```python
from build123d import *

# Parameters (mm, degrees)
F0_W     = 24
F0_H     = 24
F1_DEPTH = 120
F2_R     = 8.3
F3_DEPTH = 250
F4_W     = 28.767977
F4_H     = 14
F4_W_2   = 2.367542
F4_W_3   = 2.400435
F4_W_4   = 24
F5_DEPTH = 250


with BuildPart() as f1:
    # F0 (on Front) → F1 (new body)
    with BuildSketch(Plane.XZ):
        with Locations((-6.988064, 12)):
            Rectangle(F0_W, F0_H)
    extrude(amount=F1_DEPTH)

    # F2 (on face) → F3 (cut)
    with BuildSketch(Plane.XZ.offset(120)):
        with Locations((-6.988064, 0)):
            Circle(F2_R)
    extrude(amount=-F3_DEPTH, mode=Mode.SUBTRACT)

    # F4 (on face) → F5 (cut)
    with BuildSketch(Plane.XZ.offset(120)):
        with Locations((-7.004511, 17)):
            Rectangle(F4_W, F4_H)
        with Locations((6.195707, 17)):
            Rectangle(F4_W_2, F4_H)
        with Locations((-20.188281, 17)):
            Rectangle(F4_W_3, F4_H)
        with Locations((-6.988064, 17)):
            Rectangle(F4_W_4, F4_H)
    extrude(amount=-F5_DEPTH, mode=Mode.SUBTRACT)


solid = f1.part
```
Part model, mm, in its own coordinate system. Round coordinates to 2 decimals unless told otherwise and drop trailing zeros. Loops run counter-clockwise (first coordinate to the right, second up) from the corner with the lowest first, then second, coordinate; pieces in that order, holes last.
Item 1: Cut at B-B, the plane y = -52. Give the cut face in (x, z).
Item 2: Drill centre lines: line 1 (X direction, y = -78, z = 3.5); line 2 (X direction, y = -97.5, z = 5.5); line 3 (Z direction, x = -7.25, y = -28). Where is each one in solid material? Low to high.
Item 3: Drop a flat-ended pin along its axis: P1, Ø1.5, axis at x = -7, y = -98, coming from the -Z side. Give the stop position or say it passes through.
Item 4: Cut at A-A, the plane z = 3.75. Give the cut face in (x, y), then the cut area to 3 significant figures.
Item 5: Cut at D-D, the plane x = -11.5. Give the cut face in (y, z), then the cut area to 3 significant figures.
Item 6: Cut at C-C, the plane x = -3.5. Give the cut face in (y, z), then the cut area to 3 significant figures.
A:
1. outline: (-18.99, 0) - (-15.29, 0) arc R8.3 cw to (1.31, 0) - (5.01, 0) - (5.01, 10) - (-18.99, 10) - close
2. line 1: x = -18.99 to -14.51, 0.54 to 5.01
2. line 2: x = -18.99 to -13.2, -0.77 to 5.01
2. line 3: z = 8.3 to 10
3. P1: stops at z = 8.26
4. outline: (-18.99, -120) - (-14.39, -120) - (-14.39, 0) - (-18.99, 0) - close; (0.42, -120) - (5.01, -120) - (5.01, 0) - (0.42, 0) - close
4. area: 1,100 mm2
5. outline: (-120, 6.97) - (0, 6.97) - (0, 10) - (-120, 10) - close
5. area: 364 mm2
6. outline: (-120, 7.53) - (0, 7.53) - (0, 10) - (-120, 10) - close
6. area: 296 mm2
